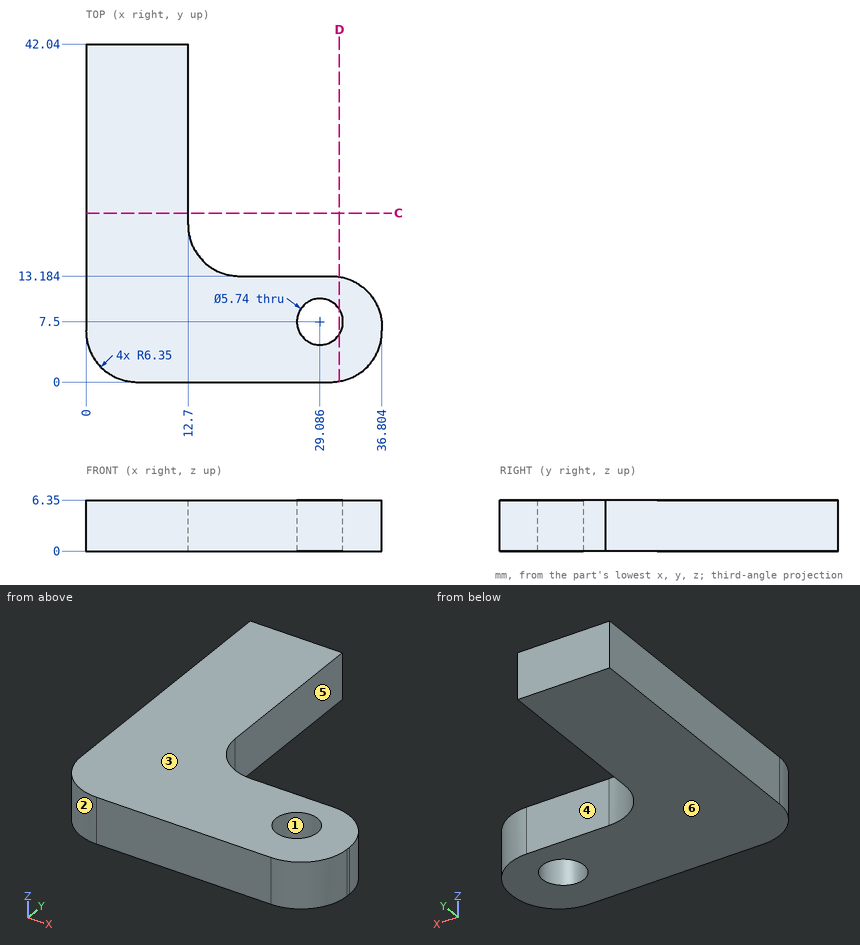
Check sheet for the drawn part. Datum: minimum x, y, z corner. Units: mm. A direction names the side the tool comes from. Round coordinates to 2 decimals unless told otherwise and drop trailing zeros. Order: outer loops, then holes, each group sorted by start corner. A loop starts at its lowest first (then second) coordinate and runs counter-clockwise, first axis right, second up. Notation, with made-up numbers: (41, -16.75) -> (86, -16.75) arc R4 ccw to (86, -9.75) -> close; hole circle Ø11 at (45, 24). An arc over 180 degrees is marked (long way). Put each result on its own line as item: value.
1) Mould release check, pull along Y, two halves, no side actions. Record for the marked faces 1, 2, 3 and 4: +Y half, -Y half, draft (parallel to the pull), parting line (faces both ways), or undercut.
Final values:
face 1: undercut
face 2: -Y half
face 3: draft
face 4: +Y half
2) Section check C-C (y = 21). Record the cut outline in (x, z).
Final values:
outline: (0, 0) -> (12.7, 0) -> (12.7, 6.35) -> (0, 6.35) -> close
3) Depth check by flat-ended pin: pin 1 (3 mm diameter, centred on y = 17.5, z = 2, fed in from +X) (1 decimal). Enter the tip coordinate at first touch or a pass-through.
Final values:
pin 1: stops at x = 13.8
4) Material ranges on line 1 (X direction, y = 28, z = 0.5); line 2 (Y direction, x = 23, z = 3) (1 decimal); line 3 (X direction, y = 10, z = 1) (1 decimal), recorded low to high.
Final values:
line 1: x = 0 to 12.7
line 2: y = 0 to 13.2
line 3: x = 0 to 27.7, 30.5 to 36
5) Section check D-D (x = 31.5). Record the cut outline in (y, z).
Final values:
outline: (0.09, 0) -> (5.95, 0) -> (5.95, 6.35) -> (0.09, 6.35) -> close; (9.05, 0) -> (13.1, 0) -> (13.1, 6.35) -> (9.05, 6.35) -> close
6) Set-up check for the marked faces 5 and 6: record each of +Z, -Z, +X, -X, +Y, -Y from which the full face is reachable in a straight line by a thin tool's end or side.
Final values:
face 5: +Z, -Z, +X, +Y
face 6: -Z, +X, -X, +Y, -Y
